The model under review builds one solid part; all positions refer to its coordinate system, in mm. A direction names the side the tool comes from. Give positions to 0.01 mm unless a question says otherwise; leave off trailing zeros. Loops run counter-clockwise (first coordinate to the right, second up) from the corner with the lowest first, then second, coordinate; pieces in that order, holes last. Notation, with made-up numbers: M 4,2.25 L 32,2.25 A28 ccw 32,33.25 Z; hole C 31.25,78 d2. An arc over 180 degrees is marked long. One line per item, written item: value. Start each with the question number.
Q1. For faces 4 (the face through (-5, 0, 168)), 5 (the face through (-30, -35, 40)), 6 (the face through (-10, -10, 168)), 7 (the face through (-5, -10, 40)), list the 3-axis set-ups (+Z, -Z, +X, -X, +Y, -Y) from which the entire face can be reached by the end or side of a thin tool; tool diameter is ignored.
Q2. For pin 1 (18 mm diameter, centred on x = -20.5, z = 220.5, fed in from +Y); pin 2 (3 mm diameter, centred on x = -2.5, y = -9.5, fed in from -Z); pin 3 (8 mm diameter, centred on x = -35, z = 19.36, fed in from +Y); pin 4 (10 mm diameter, centred on y = -9.5, z = 130.5, fed in from -X), all flat-tipped, find the tip position at first contact; note any pin that passes through.
Q3. We need section B-B on z = 122.5. Write out the cut boundary in (x, y).
Q4. To check wall thickness, follow line 1 along Z through (x, y) = (-35, -22.75); line 2 along Y through (x, z) = (-31, 189); line 3 along X through (y, z) = (-15, 253). State the ranges of each line that lie inside material, in increasing order. Write a range as from..to.
Q5. Mouldability with a two-part tool opening along Z and no side actions: class faces 1 (the face through (-38.968, -24.93, 16.322)), 2 (the face through (-36, -20, 148)), 3 (the face through (-30, -29, 300)) as released by +Z, released by -Z, zero draft, split by the parting line, or undercut.
Q6. We need section C-C on y = -33. Write out the cut boundary in (x, z).
Q7. We need section D-D on x = -56. Write out the cut boundary in (y, z), plus the area to 3 significant figures.
Q8. We need section A-A on x = -35. Write out the cut boundary in (y, z), plus the area to 3 significant figures.
```python
from build123d import *

# Parameters (mm, degrees)
EXTRUDE_1_DEPTH     = 300
SKETCH_2_W          = 10
SKETCH_2_H          = 20
CUT_EXTRUDE_1_DEPTH = 40
SKETCH_4_R          = 5
CUT_EXTRUDE_2_DEPTH = 307.594194335
CUT_EXTRUDE_3_DEPTH = 309.544972411
FILLET_1_R          = 10


with BuildPart() as part:
    # 草图1 → 凸台-拉伸1 (new body)
    with BuildSketch(Plane.XY):
        Polygon((0, 0), (0, -40), (60, -40), (60, -20), (10, -20), (10, 0), align=None)
    extrude_1 = extrude(amount=EXTRUDE_1_DEPTH)

    # 草图2 → 切除-拉伸1 (cut)
    with BuildSketch(Plane(origin=(0, 0, 0), x_dir=(-1, 0, 0), z_dir=(0, 0, -1))):
        with Locations((-5, -10)):
            Rectangle(SKETCH_2_W, SKETCH_2_H)
        Polygon((-10, -30), (0, -30), (0, -40), (-10, -40), (-60, -40), (-60, -30), align=None)
    cut_extrude_1 = extrude(amount=-CUT_EXTRUDE_1_DEPTH, mode=Mode.SUBTRACT)

    # 草图4 → 切除-拉伸2 (cut, symmetric)
    with BuildSketch(Plane(origin=(0, -20, 0), x_dir=(1, 0, 0), z_dir=(0, 1, 0))):
        with Locations(Location((35, -19.364916731, 0), (0, 0, 180))):
            Circle(SKETCH_4_R)
    cut_extrude_2 = extrude(amount=CUT_EXTRUDE_2_DEPTH, both=True, mode=Mode.SUBTRACT)

    # 镜向1: 凸台-拉伸1, 切除-拉伸1, 切除-拉伸2 across plane
    add(extrude_1.mirror(Plane(origin=(0, 0, 300), x_dir=(0, 0, 1), z_dir=(1, 0, 0))))
    add(cut_extrude_1.mirror(Plane(origin=(0, 0, 300), x_dir=(0, 0, 1), z_dir=(1, 0, 0))), mode=Mode.SUBTRACT)
    add(cut_extrude_2.mirror(Plane(origin=(0, 0, 300), x_dir=(0, 0, 1), z_dir=(1, 0, 0))), mode=Mode.SUBTRACT)

    # 草图6 → 切除-拉伸3 (cut, through all)
    with BuildSketch(Plane(origin=(0, 0, 0), x_dir=(1, 0, 0), z_dir=(0, 1, 0))):
        Polygon((0, -314.936962627), (157.439827962, -317.852514996), (163.764973114, 23.705323245), (0, 26.738007932), align=None)
    extrude(amount=-CUT_EXTRUDE_3_DEPTH, mode=Mode.SUBTRACT)

    # 圆角1
    fillet_1_edges = [part.edges().sort_by_distance(p)[0] for p in [
        (0, -25, 0),
        (-60, -25, 0),
    ]]
    fillet(fillet_1_edges, radius=FILLET_1_R)


solid = part.part
```
Solved:
1. face 4: +Z, -Z, +X, -X, +Y
1. face 5: -Z, +X, -X, -Y
1. face 6: +Z, -Z, -X, +Y
1. face 7: -Z, +X, -X, +Y
2. pin 1: y = -20
2. pin 2: z = 40
2. pin 3: through
2. pin 4: x = -10
3. outline: M -60,-40 L 0,-40 L 0,0 L -10,0 L -10,-20 L -60,-20 Z
4. line 1: 0..14.36, 24.36..300
4. line 2: -40..-20
4. line 3: -10..0
5. face 1: undercut
5. face 2: zero draft
5. face 3: released by +Z
6. outline: M -60,40 L 0,40 L 0,300 L -60,300 Z
7. outline: M -40,40 L -30,40 L -30,2 L -20,2 L -20,300 L -40,300 Z
7. area: 5,580 mm2
8. outline: M -40,40 L -30,40 L -30,24.36 L -20,24.36 L -20,300 L -40,300 Z; M -30,0 L -20,0 L -20,14.36 L -30,14.36 Z
8. area: 5,500 mm2
